from build123d import *

# Parameters (mm, degrees)
F0_W     = 57.15
F0_H     = 44.45
F1_DEPTH = 25.4
F3_R     = 12.7
F4_DEPTH = 25.401
F5_DEPTH = 12.7


with BuildPart() as f1:
    # F0 (on Front) → F1 (new body)
    with BuildSketch(Plane.XZ):
        with Locations((-28.575, 22.225)):
            Rectangle(F0_W, F0_H)
    extrude(amount=F1_DEPTH)

    # F3 (on face) → F4 (cut, through all)
    with BuildSketch(Plane.XZ.offset(25.4)):
        with Locations((-26.811862, 23.974629)):
            Circle(F3_R)
    extrude(amount=-F4_DEPTH, mode=Mode.SUBTRACT)

    # F2 (on face) → F5 (cut)
    with BuildSketch(Plane.XZ.offset(25.4)):
        Polygon((0, 44.45), (-38.1, 44.45), (-12.7, 0), (0, 0), align=None)
    extrude(amount=-F5_DEPTH, mode=Mode.SUBTRACT)


solid = f1.part
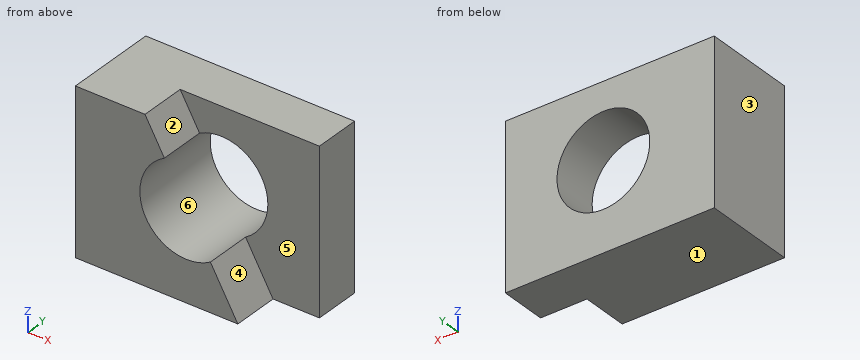
Build history of the part. All positions in model axes, mm. Face numbers are marked on the shaded views. A direction names the side the tool comes from. Coordinates: 2 decimals unless noted, no trailing zeros. Order: outer loops, then holes, each group sorted by start corner. A loop starts at its lowest first (then second) coordinate and runs counter-clockwise, first axis right, second up. Notation, with made-up numbers: (-32.75, 10) -> (10.25, 10) arc R16 cw to (10.25, 22) -> close; hole circle Ø6 at (50, 44.5). An arc over 180 degrees is marked (long way). One line per item, written item: value.
(1) Slice it at A-A, the plane x = -16.5. List the corners of the cut face in (y, z).
Checked values:
outline: (-25.4, 0) -> (0, 0) -> (0, 16.56) -> (-12.7, 16.56) -> (-12.7, 6.65) -> (-25.4, 6.65) -> close; (-12.7, 31.39) -> (0, 31.39) -> (0, 44.45) -> (-12.7, 44.45) -> close
(2) Slice it at D-D, the plane y = -7.5. List the corners of the cut face in (x, z).
Checked values:
outline: (-57.15, 0) -> (0, 0) -> (0, 44.45) -> (-57.15, 44.45) -> close; hole circle Ø25.4 at (-26.81, 23.97)
(3) Drop flat-ended pins along their axis: pin 1 Ø6 at (y, z) = (-22, 33.5) entering from +X; pin 2 Ø15 at (x, z) = (-26.81, 23.97) entering from +Y; pin 3 Ø2 at (x, z) = (-13.5, 9) entering from -Y. Give the stop position or say it passes through.
Checked values:
pin 1: x = -32.8
pin 2: through
pin 3: y = -12.7
(4) Probe line 1 (X direction, y = -7.5, z = 24.5); line 2 (Y direction, x = -16, z = 42.5); line 3 (Z direction, x = -34, y = -2.75). List the from-to ranges inside material, lowest first. Write a range as [from, to].
Checked values:
line 1: [-57.15, -39.5], [-14.12, 0]
line 2: [-12.7, 0]
line 3: [0, 13.5], [34.44, 44.45]
(5) Slice it at B-B, the plane z = 18. List the corners of the cut face in (x, y) (3 decimals).
Checked values:
outline: (-57.15, -25.4) -> (-38.019, -25.4) -> (-38.019, 0) -> (-57.15, 0) -> close; (-15.605, -12.7) -> (0, -12.7) -> (0, 0) -> (-15.605, 0) -> close
(6) Tool access for the marked faces 1 and 2: list every direction of +Z, -Z, +X, -X, +Y, -Y with a clear straight run to the whole face (end or side of a thin tool).
Checked values:
face 1: -Z, +X, -X, +Y, -Y
face 2: +Z, +X, -Y
(7) Slice it at C-C, the plane y = -14.5. List the corners of the cut face in (x, z), plus the area to 3 significant figures.
Checked values:
outline: (-57.15, 0) -> (-12.7, 0) -> (-20.2, 13.13) arc R12.7 cw (long way) to (-32.8, 35.17) -> (-38.1, 44.45) -> (-57.15, 44.45) -> close
area: 1,150 mm2
(8) Mould opens along X. For the marked faces 3, 4, 5 and 6 say: pulls with the +X half, pulls with the -X half, needs draft (parallel to the pull), parting line crosses it, or undercut.
Checked values:
face 3: pulls with the -X half
face 4: pulls with the +X half
face 5: needs draft
face 6: undercut
